```python
from build123d import *

# Parameters (mm, degrees)
F0_W              = 482.6
F0_H              = 533.2
F1_DEPTH          = 1.6
F2_W              = 16
F2_H              = 533.2
F3_DEPTH          = 1.6
F4_W              = 16
F4_H              = 533.2
F5_DEPTH          = 1.6
F6_W              = 476.6
F6_H              = 16
F7_DEPTH          = 1.6
F8_W              = 476.6
F8_H              = 16
F9_DEPTH          = 1.6
F10_W             = 381
F10_H             = 431.5
F11_DEPTH         = 1.6
F12_W             = 3.5
F12_H             = 6.8
F13_DEPTH         = 1.6
F13_COPIES3_COUNT = 2
F13_COPIES3_PITCH = 652.537999
F13_COPIES4_COUNT = 2
F13_COPIES4_PITCH = 566.888933
F14_W             = 3.5
F14_H             = 6.8
F15_DEPTH         = 1.6
F16_W             = 23.3
F16_H             = 14
F17_DEPTH         = 16


# Not quite as in the source:
# - a pattern or mirror of a feature is missing from the dataset's text; its kind, count and spacing are read off the source's solid


with BuildPart() as f1:
    # F0 (on Front) → F1 (new body)
    with BuildSketch(Plane.XZ):
        Rectangle(F0_W, F0_H)
    extrude(amount=-F1_DEPTH)

    # F2 (on face) → F3 (join)
    with BuildSketch(Plane(origin=(-241.3, 0, 0), x_dir=(0, -1, 0), z_dir=(-1, 0, 0))):
        with Locations((-8, 0)):
            Rectangle(F2_W, F2_H)
    extrude(amount=-F3_DEPTH)

    # F4 (on face) → F5 (join)
    with BuildSketch(Plane.YZ.offset(241.3)):
        with Locations((8, 0)):
            Rectangle(F4_W, F4_H)
    extrude(amount=-F5_DEPTH)

    # F6 (on face) → F7 (join)
    with BuildSketch(Plane.XY.offset(266.6)):
        with Locations((0, 8)):
            Rectangle(F6_W, F6_H)
    extrude(amount=-F7_DEPTH)

    # F8 (on face) → F9 (join)
    with BuildSketch(Plane(origin=(0, 0, -266.6), x_dir=(1, 0, 0), z_dir=(0, 0, -1))):
        with Locations((0, -8)):
            Rectangle(F8_W, F8_H)
    extrude(amount=-F9_DEPTH)

    # F10 (on face) → F11 (cut)
    with BuildSketch(Plane.XZ):
        Rectangle(F10_W, F10_H)
    extrude(amount=-F11_DEPTH, mode=Mode.SUBTRACT)

    # F12 (on face) → F13 (cut)
    with BuildSketch(Plane.XZ):
        with Locations((-232.5, -228.9)):
            Rectangle(F12_W, F12_H)
        with BuildLine():
            Line((-230.75, -225.5), (-230.75, -232.3))
            ThreePointArc((-230.75, -232.3), (-227.35, -228.9), (-230.75, -225.5))
        make_face()
        with BuildLine():
            ThreePointArc((-234.25, -225.5), (-237.65, -228.9), (-234.25, -232.3))
            Line((-234.25, -232.3), (-234.25, -225.5))
        make_face()
    f13 = extrude(amount=-F13_DEPTH, mode=Mode.SUBTRACT)

    # F13_copies: F13 across plane
    add(f13.mirror(Plane.XY), mode=Mode.SUBTRACT)

    # F13_copies1: F13 across plane
    add(f13.mirror(Plane.XY.offset(-66.775)), mode=Mode.SUBTRACT)

    # F13_copies2: F13 across plane
    add(f13.mirror(Plane(origin=(0, 0, 0), x_dir=(0, 0, 1), z_dir=(1, 0, 0))), mode=Mode.SUBTRACT)

    # F13_copies3: F13 ×2
    with Locations(*[Vector(0.7126021792, 0, 0.701568339) * (i * F13_COPIES3_PITCH) for i in range(1, F13_COPIES3_COUNT)]):
        add(f13, mode=Mode.SUBTRACT)

    # F13_copies4: F13 ×2
    with Locations(*[Vector(0.8202664981, 0, 0.5719815312) * (i * F13_COPIES4_PITCH) for i in range(1, F13_COPIES4_COUNT)]):
        add(f13, mode=Mode.SUBTRACT)

    # F14 (on face) → F15 (cut)
    with BuildSketch(Plane.XZ):
        with Locations((-232.5, -95.35)):
            Rectangle(F14_W, F14_H)
        with BuildLine():
            Line((-230.75, -91.95), (-230.75, -98.75))
            ThreePointArc((-230.75, -98.75), (-227.35, -95.35), (-230.75, -91.95))
        make_face()
        with BuildLine():
            ThreePointArc((-234.25, -91.95), (-237.65, -95.35), (-234.25, -98.75))
            Line((-234.25, -98.75), (-234.25, -91.95))
        make_face()
    f15 = extrude(amount=-F15_DEPTH, mode=Mode.SUBTRACT)

    # F15_copies: F15 across plane
    add(f15.mirror(Plane(origin=(0, 0, 0), x_dir=(0, 0, 1), z_dir=(1, 0, 0))), mode=Mode.SUBTRACT)

    # F16 (on face) → F17 (cut)
    with BuildSketch(Plane.XZ):
        with Locations((-229.65, 244.8)):
            Rectangle(F16_W, F16_H)
        with BuildLine():
            Line((-218, 251.8), (-218, 237.8))
            ThreePointArc((-218, 237.8), (-211, 244.8), (-218, 251.8))
        make_face()
    extrude(amount=-F17_DEPTH, mode=Mode.SUBTRACT)


solid = f1.part
```
Model file for the job. Use its own axes, mm. A direction names the side the tool comes from. Give positions to 0.01 mm unless a question says otherwise; leave off trailing zeros. Loops run counter-clockwise (first coordinate to the right, second up) from the corner with the lowest first, then second, coordinate; pieces in that order, holes last. Notation, with made-up numbers: (-15.75, 68.25) -> (13.25, 68.25) arc R20 ccw to (13.25, 100.25) -> close; hole circle Ø10 at (-27, 61.5). An arc over 180 degrees is marked (long way). Write each question's results on one line, items separated by ' | '.
(1) Pull direction Z, two halves, no side cores. Call faces 1 (the flat face through (210, 1.6, 4)), 2 (the flat face through (-3, 8, 266.6)), 3 (the flat face through (-241.3, 8, 259)): released by +Z, released by -Z, zero draft, split by the parting line, or undercut.
Geometry results:
face 1: undercut | face 2: released by +Z | face 3: zero draft
(2) Cut at B-B on y = 13.5. List the corners of the cut face in (x, z).
Geometry results:
outline: (-241.3, -266.6) -> (-239.7, -266.6) -> (-239.7, 237.8) -> (-241.3, 237.8) -> close; (-241.3, 251.8) -> (-239.7, 251.8) -> (-239.7, 266.6) -> (-241.3, 266.6) -> close; (-238.3, -266.6) -> (238.3, -266.6) -> (238.3, -265) -> (-238.3, -265) -> close; (-238.3, 265) -> (238.3, 265) -> (238.3, 266.6) -> (-238.3, 266.6) -> close; (239.7, -266.6) -> (241.3, -266.6) -> (241.3, 266.6) -> (239.7, 266.6) -> close
(3) Cut at D-D on x = -199. List the corners of the cut face in (y, z).
Geometry results:
outline: (0, -266.6) -> (16, -266.6) -> (16, -265) -> (1.6, -265) -> (1.6, 265) -> (16, 265) -> (16, 266.6) -> (0, 266.6) -> close
(4) Probe line 1 along X through (y, z) = (14, -6); line 2 along Z through (x, y) = (-73.5, 2); line 3 along Y through (x, z) = (-204, -52.5). List the from-to ranges inside material, lowest first.
Geometry results:
line 1: x = -241.3 to -239.7, 239.7 to 241.3 | line 2: z = -266.6 to -265, 265 to 266.6 | line 3: y = 0 to 1.6
(5) Tool access for faces 4 (the flat face through (-239.7, 9, 259)), 5 (the flat face through (-3, 9, -265)), 6 (the flat face through (241.3, 8, -4)), 7 (the flat face through (-235, 1, 237.8)): list every direction of +Z, -Z, +X, -X, +Y, -Y with a clear straight run to the whole face (end or side of a thin tool).
Geometry results:
face 4: +Z, -Z, +Y | face 5: +Y | face 6: +Z, -Z, +X, +Y, -Y | face 7: -X, +Y, -Y
(6) Cut at A-A on x = -20. List the corners of the cut face in (y, z), and give its area (3 significant figures).
Geometry results:
outline: (0, -266.6) -> (16, -266.6) -> (16, -265) -> (1.6, -265) -> (1.6, -215.75) -> (0, -215.75) -> close; (0, 215.75) -> (1.6, 215.75) -> (1.6, 265) -> (16, 265) -> (16, 266.6) -> (0, 266.6) -> close | area: 209 mm²
(7) Cut at C-C on z = -195. List the corners of the cut face in (x, y), and give its area (3 significant figures).
Geometry results:
outline: (-241.3, 0) -> (-190.5, 0) -> (-190.5, 1.6) -> (-239.7, 1.6) -> (-239.7, 16) -> (-241.3, 16) -> close; (190.5, 0) -> (241.3, 0) -> (241.3, 16) -> (239.7, 16) -> (239.7, 1.6) -> (190.5, 1.6) -> close | area: 209 mm²
